from build123d import *

# Parameters (mm, degrees)
F0_W     = 12
F0_H     = 25
F1_DEPTH = 5
F2_R     = 2.5
F3_DEPTH = 5.001
F4_R     = 4.99
F5_DEPTH = 15


with BuildPart() as f1:
    # F0 (on Front) → F1 (new body)
    with BuildSketch(Plane.XZ):
        with Locations((6, 12.5)):
            Rectangle(F0_W, F0_H)
    extrude(amount=F1_DEPTH)

    # F2 (on face) → F3 (cut, through all)
    with BuildSketch(Plane.XZ.offset(5)):
        with Locations((6, 4)):
            Circle(F2_R)
    extrude(amount=-F3_DEPTH, mode=Mode.SUBTRACT)

    # F4 (on face) → F5 (join)
    with BuildSketch(Plane.XZ.offset(5)):
        with Locations((6, 19)):
            Circle(F4_R)
    extrude(amount=F5_DEPTH)


solid = f1.part
Build history of the part. All positions in model axes, mm. Round coordinates to 2 decimals unless told otherwise and drop trailing zeros. Loops run counter-clockwise (first coordinate to the right, second up) from the corner with the lowest first, then second, coordinate; pieces in that order, holes last. Notation, with made-up numbers: (31.5, 24.5) -> (39.5, 24.5) arc R26 cw to (39.5, 50.5) -> close; hole circle Ø1 at (-20, 21). An arc over 180 degrees is marked (long way). Use CSV: the item, a comma, the result in double quotes. Start each with the question number.
Q1. Saw through at D-D on x = 4. Give the cut face in (y, z), and give its area (3 significant figures).
Q2. Saw through at B-B on x = 6. Give the cut face in (y, z).
Q3. Saw through at A-A on z = 4. Give the cut face in (x, y).
Q4. Saw through at C-C on z = 19. Give the cut face in (x, y), and give its area (3 significant figures).
Q5. Drill centre lines: L1, parallel to Z at x = 6, y = -1.75; L2, parallel to Y at x = 11, z = 8; L3, parallel to X at y = -2.25, z = 6.25. Where is each one in solid material? Low to high.
Q6. Mould opens along Z. For faces 1 (the face through (6, 0, 13)), 2 (the face through (6, -2, 25)), 3 (the face through (8.385, -2.535, 4.751)), 4 (the face through (4.92, -12.4, 14.13)) say: +Z half, -Z half, draft (parallel to the pull), parting line (faces both ways), or undercut.
Q7. Flat gauge pins, fed straight in: pin 1 Ø5 at (x, y) = (4.5, -12) entering from -Z; pin 2 Ø5 at (y, z) = (-16.5, 15) entering from +X; pin 3 Ø3 at (y, z) = (-8.5, 14) entering from -X. Where does each tip first touch, or does it go through?
Solutions:
1,outline,"(-20, 14.43) -> (-5, 14.43) -> (-5, 5.5) -> (0, 5.5) -> (0, 25) -> (-5, 25) -> (-5, 23.57) -> (-20, 23.57) -> close; (-5, 0) -> (0, 0) -> (0, 2.5) -> (-5, 2.5) -> close"
1,area,"247 mm^2"
2,outline,"(-20, 14.01) -> (-5, 14.01) -> (-5, 6.5) -> (0, 6.5) -> (0, 25) -> (-5, 25) -> (-5, 23.99) -> (-20, 23.99) -> close; (-5, 0) -> (0, 0) -> (0, 1.5) -> (-5, 1.5) -> close"
3,outline,"(0, -5) -> (3.5, -5) -> (3.5, 0) -> (0, 0) -> close; (8.5, -5) -> (12, -5) -> (12, 0) -> (8.5, 0) -> close"
4,outline,"(0, -5) -> (1.01, -5) -> (1.01, -20) -> (10.99, -20) -> (10.99, -5) -> (12, -5) -> (12, 0) -> (0, 0) -> close"
4,area,"210 mm^2"
5,L1,"z = 0 to 1.5, 6.5 to 25"
5,L2,"y = -5 to 0"
5,L3,"x = 0 to 4.91, 7.09 to 12"
6,face 1,"draft"
6,face 2,"+Z half"
6,face 3,"undercut"
6,face 4,"parting line"
7,pin 1,"stops at z = 14.01"
7,pin 2,"stops at x = 10.76"
7,pin 3,"stops at x = 2.44"
